Source: CAD feature listing. Evaluate the final solid. Frame: model axes, mm. A direction names the side the tool comes from. Coordinates: 2 decimals unless noted, no trailing zeros. Order: outer loops, then holes, each group sorted by start corner. A loop starts at its lowest first (then second) coordinate and runs counter-clockwise, first axis right, second up. Notation, with made-up numbers: (88, -5.75) - (93, -5.75) arc R13 cw to (93, 2.25) - close; hole circle Ø2 at (82.5, -32). An arc over 180 degrees is marked (long way). One line per question, with ' | ' between items. Start each with the question number.
(1) Section D-D (y = 17). Return the cut outline in (x, z), then the cut area to 3 significant figures.
(2) Line query: line 1 along Y through (x, z) = (-56.5, 16.45); line 2 along Y through (x, z) = (-10, 14.5); line 3 along Z through (x, y) = (-48, 15.5). Output: solid intervals per line, ascending.
(3) Access query for faces 1 (the flat face through (-26, 33, 20)), 2 (the flat face through (-53, 26, 15)). Directions: +Z, -Z, +X, -X, +Y, -Y. A direction counts if a zero-diameter tool reaches every point of the face in a straight line with its end or side. Return the directions, or none.
(4) Section A-A (y = 29). Return the cut outline in (x, z), then the cut area to 3 significant figures.
(5) Section B-B (x = -25.5). Return the cut outline in (y, z).
(6) Draft query along X for faces 3 (the cylindrical face through (-54.831, 17.526, 17.465)), 4 (the flat face through (-18, 65, 12)), 5 (the flat face through (-65, 32, 17)). Return one class per face: +X half, -X half, draft (parallel to the pull), parting line (faces both ways), or undercut.
(7) Contact query for flat-ended pins moving along their axis: P1, Ø1.5, axis at x = -27, y = 8, coming from the -Z side; P2, Ø3, axis at y = 35.5, z = 12.5, coming from the -X side; P3, Ø3.5, axis at x = -10, y = 17, coming from the -Z side. Output: stop coordinate, or through.
(8) Section C-C (x = -41). Return the cut outline in (y, z).
from build123d import *

# Parameters (mm, degrees)
F0_W     = 19
F0_H     = 65
F0_R     = 2.75
F0_W_2   = 46
F0_R_2   = 1.75
F0_R_3   = 12.5
F1_DEPTH = 20
F2_DEPTH = 15


with BuildPart() as f1:
    # F0 (on Top) → F1 (new body)
    with BuildSketch(Plane.XY):
        with Locations((-9.5, 32.5)):
            Rectangle(F0_W, F0_H)
        with Locations((-10, 17)):
            Circle(F0_R, mode=Mode.SUBTRACT)
        with Locations((-10, 48)):
            Circle(F0_R, mode=Mode.SUBTRACT)
        with Locations((-42, 32.5)):
            Rectangle(F0_W_2, F0_H)
        with Locations((-56.5, 17)):
            Circle(F0_R_2, mode=Mode.SUBTRACT)
        with Locations((-25.5, 17)):
            Circle(F0_R_2, mode=Mode.SUBTRACT)
        with Locations((-56.5, 48)):
            Circle(F0_R_2, mode=Mode.SUBTRACT)
        with Locations((-41, 32.5)):
            Circle(F0_R_3, mode=Mode.SUBTRACT)
        with Locations((-25.5, 48)):
            Circle(F0_R_2, mode=Mode.SUBTRACT)
    extrude(amount=F1_DEPTH)

    # F0 (on Top) → F2 (cut)
    with BuildSketch(Plane.XY):
        with Locations((-42, 32.5)):
            Rectangle(F0_W_2, F0_H)
        with Locations((-56.5, 17)):
            Circle(F0_R_2, mode=Mode.SUBTRACT)
        with Locations((-25.5, 17)):
            Circle(F0_R_2, mode=Mode.SUBTRACT)
        with Locations((-56.5, 48)):
            Circle(F0_R_2, mode=Mode.SUBTRACT)
        with Locations((-41, 32.5)):
            Circle(F0_R_3, mode=Mode.SUBTRACT)
        with Locations((-25.5, 48)):
            Circle(F0_R_2, mode=Mode.SUBTRACT)
    extrude(amount=F2_DEPTH, mode=Mode.SUBTRACT)


solid = f1.part
Response values:
1) outline: (-65, 15) - (-58.25, 15) - (-58.25, 20) - (-65, 20) - close; (-54.75, 15) - (-27.25, 15) - (-27.25, 20) - (-54.75, 20) - close; (-23.75, 15) - (-19, 15) - (-19, 0) - (-12.75, 0) - (-12.75, 20) - (-23.75, 20) - close; (-7.25, 0) - (0, 0) - (0, 20) - (-7.25, 20) - close | area: 465 mm²
2) line 1: y = 0 to 15.25, 18.75 to 46.25, 49.75 to 65 | line 2: y = 0 to 14.25, 19.75 to 45.25, 50.75 to 65 | line 3: z = 15 to 20
3) face 1: +Z, +X, -X, +Y, -Y | face 2: -Z, -X, +Y, -Y
4) outline: (-65, 15) - (-53, 15) - (-53, 20) - (-65, 20) - close; (-29, 15) - (-19, 15) - (-19, 0) - (0, 0) - (0, 20) - (-29, 20) - close | area: 490 mm²
5) outline: (0, 15) - (15.25, 15) - (15.25, 20) - (0, 20) - close; (18.75, 15) - (46.25, 15) - (46.25, 20) - (18.75, 20) - close; (49.75, 15) - (65, 15) - (65, 20) - (49.75, 20) - close
6) face 3: undercut | face 4: draft | face 5: -X half
7) P1: stops at z = 15 | P2: stops at x = -19 | P3: passes through
8) outline: (0, 15) - (20, 15) - (20, 20) - (0, 20) - close; (45, 15) - (65, 15) - (65, 20) - (45, 20) - close
